from build123d import *

# Parameters (mm, degrees)
SKETCH_1_R      = 1
EXTRUDE_1_DEPTH = 2


with BuildPart() as part:
    # 草圖1 → 填料-伸長1 (new body)
    with BuildSketch(Plane.XY):
        with BuildLine():
            Line((-28.161562759, 19.347959184), (-29.161562759, 19.347959184))
            Line((-29.161562759, 19.347959184), (-29.161562759, 18.347959184))
            Line((-29.161562759, 18.347959184), (-29.161562759, 12.847959184))
            ThreePointArc((-29.161562759, 12.847959184), (-28.161562759, 11.847959184), (-29.161562759, 10.847959184))
            Line((-29.161562759, 10.847959184), (-31.161562759, 10.847959184))
            Line((-31.161562759, 10.847959184), (-31.161562759, 6.847959184))
            Line((-31.161562759, 6.847959184), (-29.161562759, 6.847959184))
            ThreePointArc((-29.161562759, 6.847959184), (-28.161562759, 5.847959184), (-29.161562759, 4.847959184))
            Line((-29.161562759, 4.847959184), (-29.161562759, 0.847959184))
            ThreePointArc((-29.161562759, 0.847959184), (-28.161562759, -0.152040816), (-29.161562759, -1.152040816))
            Line((-29.161562759, -1.152040816), (-31.161562759, -1.152040816))
            Line((-31.161562759, -1.152040816), (-31.161562759, -5.152040816))
            Line((-31.161562759, -5.152040816), (-29.161562759, -5.152040816))
            ThreePointArc((-29.161562759, -5.152040816), (-28.161562759, -6.152040816), (-29.161562759, -7.152040816))
            Line((-29.161562759, -7.152040816), (-29.161562759, -12.652040816))
            Line((-29.161562759, -12.652040816), (-29.161562759, -13.652040816))
            Line((-29.161562759, -13.652040816), (-28.161562759, -13.652040816))
            Line((-28.161562759, -13.652040816), (23.438437241, -13.652040816))
            Line((23.438437241, -13.652040816), (24.438437241, -13.652040816))
            Line((24.438437241, -13.652040816), (24.438437241, -12.652040816))
            Line((24.438437241, -12.652040816), (24.438437241, -7.152040816))
            ThreePointArc((24.438437241, -7.152040816), (23.438437241, -6.152040816), (24.438437241, -5.152040816))
            Line((24.438437241, -5.152040816), (26.438437241, -5.152040816))
            Line((26.438437241, -5.152040816), (26.438437241, -1.152040816))
            Line((26.438437241, -1.152040816), (24.438437241, -1.152040816))
            ThreePointArc((24.438437241, -1.152040816), (23.438437241, -0.152040816), (24.438437241, 0.847959184))
            Line((24.438437241, 0.847959184), (24.438437241, 4.847959184))
            ThreePointArc((24.438437241, 4.847959184), (23.438437241, 5.847959184), (24.438437241, 6.847959184))
            Line((24.438437241, 6.847959184), (26.438437241, 6.847959184))
            Line((26.438437241, 6.847959184), (26.438437241, 10.847959184))
            Line((26.438437241, 10.847959184), (24.438437241, 10.847959184))
            ThreePointArc((24.438437241, 10.847959184), (23.438437241, 11.847959184), (24.438437241, 12.847959184))
            Line((24.438437241, 12.847959184), (24.438437241, 18.347959184))
            Line((24.438437241, 18.347959184), (24.438437241, 19.347959184))
            Line((24.438437241, 19.347959184), (23.438437241, 19.347959184))
            Line((23.438437241, 19.347959184), (-28.161562759, 19.347959184))
        make_face()
        with Locations((22.438437241, 8.847959184)):
            Circle(SKETCH_1_R, mode=Mode.SUBTRACT)
        with Locations((-27.161562759, 8.847959184)):
            Circle(SKETCH_1_R, mode=Mode.SUBTRACT)
        with Locations((-27.161562759, -3.152040816)):
            Circle(SKETCH_1_R, mode=Mode.SUBTRACT)
        with Locations((22.438437241, -3.152040816)):
            Circle(SKETCH_1_R, mode=Mode.SUBTRACT)
    extrude(amount=EXTRUDE_1_DEPTH)


solid = part.part
The listing builds one solid part. Answer for the finished solid, in the listing's coordinates (mm). A direction names the side the tool comes from. Give positions to 0.01 mm unless a question says otherwise; leave off trailing zeros. Write each loop counter-clockwise with the first axis right and the second up, starting at its lowest first coordinate (ties: lowest second). Pieces come first, ordered by that corner, then holes. Notation, with made-up numbers: (-21, 32) - (35, 32) arc R22 ccw to (35, 70) - close; hole circle Ø2 at (54, -23). An arc over 180 degrees is marked (long way). Use a Markdown table: item, result.
1. A tool of negligible diameter and unlimited length cuts with its end or side. For faces 1 (the flat face through (-30, -1.152, 1)), 2 (the flat face through (-29.162, -10, 1)), 3 (the flat face through (25, -1.152, 1)), 4 (the flat face through (25, -5.152, 1)), from which of +Z, -Z, +X, -X, +Y, -Y can it reach the whole face along a straight path? Write none if from no direction.
Values follow:
| item | result |
|---|---|
| face 1 | +Z, -Z, -X |
| face 2 | +Z, -Z, -X, -Y |
| face 3 | +Z, -Z, +X |
| face 4 | +Z, -Z, +X, -Y |
2. Section B-B on x = 22 is taken. Write down the section's boundary in (y, z).
Values follow:
| item | result |
|---|---|
| outline | (-13.65, 0) - (-4.05, 0) - (-4.05, 2) - (-13.65, 2) - close; (-2.25, 0) - (7.95, 0) - (7.95, 2) - (-2.25, 2) - close; (9.75, 0) - (19.35, 0) - (19.35, 2) - (9.75, 2) - close |
3. For a pull along X with two mould halves and no side action, classify faces 5 (the flat face through (-2, 19.348, 1)), 6 (the cylindrical face through (23.44, -0.17, 0.99)), 7 (the flat face through (-31.162, -3, 1)), 8 (the cylindrical face through (-26.21, -2.85, 0.99)) as released by +X, released by -X, zero draft, split by the parting line, or undercut.
Values follow:
| item | result |
|---|---|
| face 5 | zero draft |
| face 6 | released by +X |
| face 7 | released by -X |
| face 8 | undercut |
4. Section A-A on z = 1.7 is taken. Count the separate pieces of the cut face and the enclosed holes in it, plus the area to 3 significant figures.
Values follow:
| item | result |
|---|---|
| separate pieces | 1 |
| enclosed holes | 4 |
| area | 1,780 mm² |
5. Each of these flat-tipped pins is pushed along its axis until it touches: P1, Ø0.6, axis at x = 25.5, z = 1, coming from the +Y side; P2, Ø1.6, axis at x = -27.16, y = -3.15, coming from the -Z side; P3, Ø1, axis at x = -30, z = 1, coming from the -Y side; P4, Ø0.6, axis at y = 17.5, z = 1, coming from the +X side. Where does it stop, or does it pass through?
Values follow:
| item | result |
|---|---|
| P1 | stops at y = 10.85 |
| P2 | passes through |
| P3 | stops at y = -5.15 |
| P4 | stops at x = 24.44 |
6. Section C-C on y = -9 is taken. Write down the section's boundary in (x, z), plus the area to 3 significant figures.
Values follow:
| item | result |
|---|---|
| outline | (-29.16, 0) - (24.44, 0) - (24.44, 2) - (-29.16, 2) - close |
| area | 107 mm² |
7. Find the intervals of material crossed by probe 1 along X at (y, z) = (-3.5, 1.55); probe 2 along X at (y, z) = (8, 0.6); probe 3 along Y at (x, z) = (23, 0.8), in increasing order. Write a range as from..to.
Values follow:
| item | result |
|---|---|
| probe 1 | x = -31.16..-28.1, -26.22..21.5, 23.38..26.44 |
| probe 2 | x = -31.16..-27.69, -26.63..21.91, 22.97..26.44 |
| probe 3 | y = -13.65..-3.98, -2.32..8.02, 9.68..19.35 |
